from build123d import *

# Parameters (mm, degrees)
F0_R      = 12.7
F0_R_2    = 1.25
F1_DEPTH  = 19.05
F2_R      = 11.1125
F3_DEPTH  = 1.3335
F4_R      = 8.9535
F5_DEPTH  = 1.5875
F6_R      = 2.3876
F6_R_2    = 1.25
F7_DEPTH  = 0.8382
F9_DEPTH  = 6.5532
F10_R     = 2.0193
F11_DEPTH = 12.7
F12_R     = 5.55625
F13_DEPTH = 3.175
F15_W     = 32.121103
F15_H     = 6.35
F16_DEPTH = 25.4
F18_W     = 29.637642
F18_H     = 6.35
F19_DEPTH = 25.4


with BuildPart() as f1:
    # F0 (on Top) → F1 (new body)
    with BuildSketch(Plane.XY):
        Circle(F0_R)
        with Locations((-7.62, 0)):
            Circle(F0_R_2, mode=Mode.SUBTRACT)
        with Locations((7.62, 0)):
            Circle(F0_R_2, mode=Mode.SUBTRACT)
    extrude(amount=F1_DEPTH)

    # F2 (on face) → F3 (cut)
    with BuildSketch(Plane.XY.offset(19.05)):
        Circle(F2_R)
    extrude(amount=-F3_DEPTH, mode=Mode.SUBTRACT)

    # F4 (on face) → F5 (cut)
    with BuildSketch(Plane.XY.offset(17.7165)):
        Circle(F4_R)
    extrude(amount=-F5_DEPTH, mode=Mode.SUBTRACT)

    # F6 (on face) → F7 (cut)
    with BuildSketch(Plane(origin=(0, 0, 0), x_dir=(1, 0, 0), z_dir=(0, 0, -1))):
        with Locations((-7.62, 0)):
            Circle(F6_R)
        with Locations((-7.62, 0)):
            Circle(F6_R_2, mode=Mode.SUBTRACT)
        with Locations((7.62, 0)):
            Circle(F6_R)
        with Locations((7.62, 0)):
            Circle(F6_R_2, mode=Mode.SUBTRACT)
    extrude(amount=-F7_DEPTH, mode=Mode.SUBTRACT)

    # F8 (on face) → F9 (join)
    with BuildSketch(Plane(origin=(0, 0, 0), x_dir=(1, 0, 0), z_dir=(0, 0, -1))):
        with BuildLine():
            Line((-4.5212, 3.062886), (-4.519813, -3.064932))
            ThreePointArc((-4.519813, -3.064932), (0, -5.461), (4.519813, -3.064932))
            Line((4.519813, -3.064932), (4.5212, 3.062886))
            ThreePointArc((4.5212, 3.062886), (0, 5.461), (-4.5212, 3.062886))
        make_face()
    extrude(amount=F9_DEPTH)

    # F10 (on face) → F11 (cut)
    with BuildSketch(Plane.XY.offset(16.129)):
        Circle(F10_R)
    extrude(amount=-F11_DEPTH, mode=Mode.SUBTRACT)

    # F12 (on face) → F13 (cut)
    with BuildSketch(Plane.XY.offset(16.129)):
        Circle(F12_R)
    extrude(amount=-F13_DEPTH, mode=Mode.SUBTRACT)

    # F15 (on offset) → F16 (cut)
    with BuildSketch(Plane.XZ.offset(5.461)):
        with Locations((-0.362548, 3.175)):
            Rectangle(F15_W, F15_H)
    extrude(amount=F16_DEPTH, mode=Mode.SUBTRACT)

    # F18 (on offset) → F19 (cut)
    with BuildSketch(Plane.XZ.offset(-5.461)):
        with Locations((-0.89105, 3.175)):
            Rectangle(F18_W, F18_H)
    extrude(amount=-F19_DEPTH, mode=Mode.SUBTRACT)


solid = f1.part
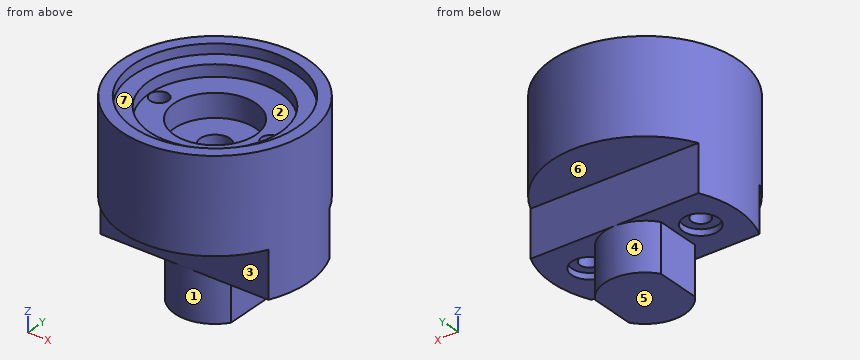
Verification items for the finished model (mm, model axes). Face numbers are marked on the shaded views. A direction names the side the tool comes from. Coordinates: 2 decimals unless noted, no trailing zeros. Order: outer loops, then holes, each group sorted by start corner. A loop starts at its lowest first (then second) coordinate and runs counter-clockwise, first axis right, second up. Notation, with made-up numbers: (-32.5, -39.75) -> (-15.5, -39.75) arc R25 cw to (-15.5, -21.75) -> close; hole circle Ø4 at (58.5, 67.25). An arc over 180 degrees is marked (long way). Use CSV: the item, a comma, the result in double quotes. Start each with the question number.
Q1. Section check C-C, the plane x = 1. Record the cut outline in (y, z).
Q2. Tool access check on the marked faces 4, 5, 6 and 7. Record the directions out of +Z, -Z, +X, -X, +Y, -Y that give a thin tool (end or side, any length) a straight path to the whole face; none if there is none.
Q3. Section check B-B, the plane z = 14.75. Record the cut outline in (x, y), and give its area (3 significant figures).
Q4. Section check D-D, the plane z = -2.25. Record the cut outline in (x, y), and give its area (3 significant figures).
Q5. Thickness scan on line 1 along Y through (x, z) = (7.62, 0.2); line 2 along Y through (x, z) = (0, 18.8); line 3 along Z through (x, y) = (6, 5.5). Record the ranges inside material, lowest first.
Q6. Depth check by flat-ended pin: P1, Ø1.8, axis at y = -1, z = -4.5, coming from the +X side; P2, Ø6, axis at x = 3.5, y = 7.5, coming from the -Z side; P3, Ø4, axis at x = -7, y = -10, coming from the -Z side; P4, Ø3, axis at x = -7.5, z = 4, coming from the +Y side. Enter the tip coordinate at first touch or a pass-through.
Q7. Draft check along X on the marked faces 1, 2 and 3. Enter one of: +X half, -X half, draft (parallel to the pull), parting line (faces both ways), or undercut.
Q8. Section check A-A, the plane x = 7.5. Record the cut outline in (y, z), and give its area (3 significant figures).
Returned:
1,outline,"(-12.66, 6.35) -> (-5.46, 6.35) -> (-5.46, 0) -> (-5.37, 0) -> (-5.37, -6.55) -> (5.37, -6.55) -> (5.37, 0) -> (5.46, 0) -> (5.46, 6.35) -> (12.66, 6.35) -> (12.66, 19.05) -> (11.07, 19.05) -> (11.07, 17.72) -> (8.9, 17.72) -> (8.9, 16.13) -> (5.47, 16.13) -> (5.47, 12.95) -> (1.75, 12.95) -> (1.75, 3.43) -> (-1.75, 3.43) -> (-1.75, 12.95) -> (-5.47, 12.95) -> (-5.47, 16.13) -> (-8.9, 16.13) -> (-8.9, 17.72) -> (-11.07, 17.72) -> (-11.07, 19.05) -> (-12.66, 19.05) -> close"
2,face 4,"-Z, +Y"
2,face 5,"-Z, +X, -X, +Y, -Y"
2,face 6,"-Z, +X, -X, +Y"
2,face 7,"+Z"
3,outline,"circle Ø25.4 at (0, 0); hole circle Ø2.5 at (-7.62, 0); hole circle Ø11.11 at (0, 0); hole circle Ø2.5 at (7.62, 0)"
3,area,"400 mm^2"
4,outline,"(-4.52, -3.06) arc R5.46 ccw to (4.52, -3.06) -> (4.52, 3.06) arc R5.46 ccw to (-4.52, 3.06) -> close"
4,area,"85.9 mm^2"
5,line 1,"y = -5.46 to -2.39, 2.39 to 5.46"
5,line 2,"y = -12.7 to -11.11, 11.11 to 12.7"
5,line 3,"z = 6.35 to 16.13"
6,P1,"stops at x = 4.52"
6,P2,"stops at z = -6.55"
6,P3,"stops at z = 6.35"
6,P4,"stops at y = 5.46"
7,face 1,"parting line"
7,face 2,"undercut"
7,face 3,"draft"
8,outline,"(-10.25, 6.35) -> (-5.46, 6.35) -> (-5.46, 0) -> (-2.38, 0) -> (-2.38, 0.84) -> (-1.24, 0.84) -> (-1.24, 16.13) -> (-4.89, 16.13) -> (-4.89, 17.72) -> (-8.2, 17.72) -> (-8.2, 19.05) -> (-10.25, 19.05) -> close; (1.24, 0.84) -> (2.38, 0.84) -> (2.38, 0) -> (5.46, 0) -> (5.46, 6.35) -> (10.25, 6.35) -> (10.25, 19.05) -> (8.2, 19.05) -> (8.2, 17.72) -> (4.89, 17.72) -> (4.89, 16.13) -> (1.24, 16.13) -> close"
8,area,"250 mm^2"
